Answer from the drawing. Dimensions are ordinates in mm from the lowest x, y and z of the part. A direction names the side the tool comes from. Round coordinates to 2 decimals unless told otherwise and drop trailing zeros. Order: outer loops, then holes, each group sorted by start corner. A loop starts at its lowest first (then second) coordinate and runs counter-clockwise, first axis right, second up.
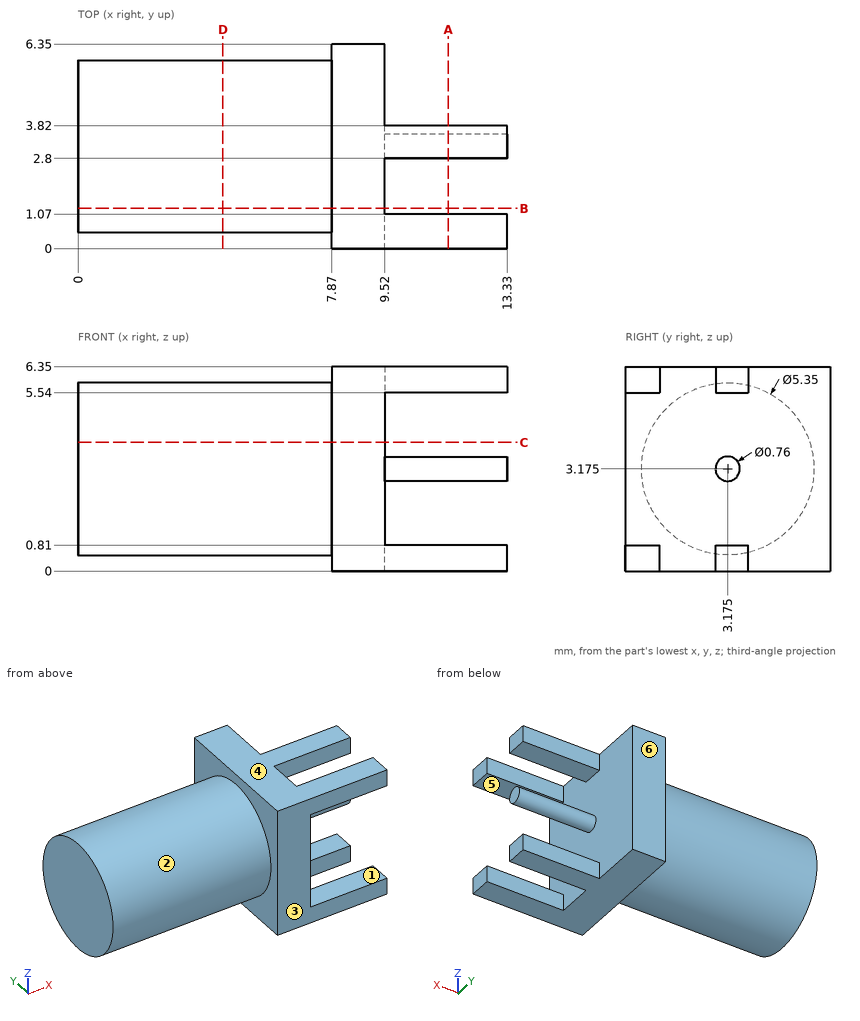
Q1. For the marked faces 1, 2 and 3, determine the directions among +Z, -Z, +X, -X, +Y, -Y from which every point of the face is accessible in a straight line to the end or side of a thin tool.
Outcome:
face 1: +X, +Y, -Y
face 2: -X
face 3: +Z, -Z, +X, -X, -Y
Q2. A cutting plane is placed at B-B, the plane y = 1.25. Give the vertices of the cut face in (x, z), plus the area to 3 significant figures.
Outcome:
outline: (0, 1.32) - (7.87, 1.32) - (7.87, 0) - (9.52, 0) - (9.52, 6.35) - (7.87, 6.35) - (7.87, 5.03) - (0, 5.03) - close
area: 39.7 mm2
Q3. For a pull along Z with two mould halves and no side action, classify the marked faces 4, 5 and 6 as released by +Z, released by -Z, zero draft, split by the parting line, or undercut.
Outcome:
face 4: released by +Z
face 5: undercut
face 6: zero draft
Q4. Straight lines are drawn through the part: probe 1 along Z at (x, y) = (10.5, 0.5); probe 2 along X at (y, z) = (6, 1); probe 3 along X at (y, z) = (2, 2.25). For each, find the intervals that lie inside material, in ascending order.
Outcome:
probe 1: z = 0 to 0.81, 5.54 to 6.35
probe 2: x = 7.87 to 9.52
probe 3: x = 0 to 9.52
Q5. Flat-ended cylindrical pins translate along their axes: pin 1 (0.6 mm diameter, centred on x = 11.5, z = 6, fed in from +Y); pin 2 (3 mm diameter, centred on x = 5, z = 1.5, fed in from -Y); pin 3 (2 mm diameter, centred on x = 5, y = 4, fed in from -Z). Find the tip coordinate at first contact, or state that the pin passes through.
Outcome:
pin 1: stops at y = 3.82
pin 2: stops at y = 0.51
pin 3: stops at z = 0.5
Q6. A cutting plane is placed at A-A, the plane x = 11.5. Give the vertices of the cut face in (y, z) (3 decimals).
Outcome:
outline: (0, 0) - (1.07, 0) - (1.07, 0.81) - (0, 0.81) - close; (0, 5.54) - (1.07, 5.54) - (1.07, 6.35) - (0, 6.35) - close; circle Ø0.76 at (3.175, 3.175); (2.8, 0) - (3.82, 0) - (3.82, 0.81) - (2.8, 0.81) - close; (2.8, 5.54) - (3.82, 5.54) - (3.82, 6.35) - (2.8, 6.35) - close
Q7. A cutting plane is placed at D-D, the plane x = 4.5. Give the vertices of the cut face in (y, z) (3 decimals), plus the area to 3 significant figures.
Outcome:
outline: circle Ø5.35 at (3.175, 3.175)
area: 22.5 mm2
Q8. A cutting plane is placed at C-C, the plane z = 4. Give the vertices of the cut face in (x, y), plus the area to 3 significant figures.
Outcome:
outline: (0, 0.63) - (7.87, 0.63) - (7.87, 0) - (9.52, 0) - (9.52, 6.35) - (7.87, 6.35) - (7.87, 5.72) - (0, 5.72) - close
area: 50.5 mm2
